from build123d import *

# Parameters (mm, degrees)
SKETCH1_W           = 22
SKETCH1_H           = 20
BOSS_EXTRUDE1_DEPTH = 18
SKETCH2_W           = 12
SKETCH2_H           = 8
CUT_EXTRUDE1_DEPTH  = 15
SKETCH3_W           = 18
SKETCH3_H           = 5
BOSS_EXTRUDE2_DEPTH = 2
LPATTERN1_COUNT     = 6
LPATTERN1_PITCH     = 24
SKETCH4_W           = 18
SKETCH4_H           = 15
BOSS_EXTRUDE3_DEPTH = 2
SKETCH5_W           = 18
SKETCH5_H           = 20
BOSS_EXTRUDE4_DEPTH = 2
SKETCH6_W           = 132
SKETCH6_H           = 2
CUT_EXTRUDE2_DEPTH  = 2
SKETCH7_W           = 146
SKETCH7_H           = 18
BOSS_EXTRUDE5_DEPTH = 6


with BuildPart() as part:
    # Sketch1 → Boss-Extrude1 (new body)
    with BuildSketch(Plane.XY):
        with Locations((11, 10)):
            Rectangle(SKETCH1_W, SKETCH1_H)
    extrude(amount=BOSS_EXTRUDE1_DEPTH)

    # Sketch2 → Cut-Extrude1 (cut)
    with BuildSketch(Plane.XZ):
        with Locations((11, 9)):
            Rectangle(SKETCH2_W, SKETCH2_H)
    extrude(amount=-CUT_EXTRUDE1_DEPTH, mode=Mode.SUBTRACT)

    # Sketch3 → Boss-Extrude2 (add)
    with BuildSketch(Plane(origin=(22, 0, 0), x_dir=(0, 0, -1), z_dir=(1, 0, 0))):
        with Locations((-9, 2.5)):
            Rectangle(SKETCH3_W, SKETCH3_H)
    extrude(amount=BOSS_EXTRUDE2_DEPTH)


with BuildPart() as lpattern1_1:
    # LPattern1: pattern copy
    add(part.part.moved(Location(Vector(1, 0, 0) * (1 * LPATTERN1_PITCH))))


with BuildPart() as lpattern1_2:
    # LPattern1: pattern copy
    add(part.part.moved(Location(Vector(1, 0, 0) * (2 * LPATTERN1_PITCH))))


with BuildPart() as lpattern1_3:
    # LPattern1: pattern copy
    add(part.part.moved(Location(Vector(1, 0, 0) * (3 * LPATTERN1_PITCH))))


with BuildPart() as lpattern1_4:
    # LPattern1: pattern copy
    add(part.part.moved(Location(Vector(1, 0, 0) * (4 * LPATTERN1_PITCH))))


with BuildPart() as lpattern1_5:
    # LPattern1: pattern copy
    add(part.part.moved(Location(Vector(1, 0, 0) * (5 * LPATTERN1_PITCH))))


with BuildPart() as lpattern1_2_1:
    add(lpattern1_2.part)

    # Combine1: union part, LPattern1_3, LPattern1_4, LPattern1_5, LPattern1_1
    add(part.part)
    add(lpattern1_3.part)
    add(lpattern1_4.part)
    add(lpattern1_5.part)
    add(lpattern1_1.part)

    # Sketch4 → Boss-Extrude3 (add)
    with BuildSketch(Plane(origin=(142, 0, 0), x_dir=(0, 0, -1), z_dir=(1, 0, 0))):
        with Locations((-9, 12.5)):
            Rectangle(SKETCH4_W, SKETCH4_H)
    extrude(amount=BOSS_EXTRUDE3_DEPTH)

    # Sketch5 → Boss-Extrude4 (add)
    with BuildSketch(Plane.ZY):
        with Locations((9, 10)):
            Rectangle(SKETCH5_W, SKETCH5_H)
    extrude(amount=BOSS_EXTRUDE4_DEPTH)

    # Sketch6 → Cut-Extrude2 (cut)
    with BuildSketch(Plane(origin=(0, 0, 0), x_dir=(-1, 0, 0), z_dir=(0, -1, 0))):
        with Locations((-71, -9)):
            Rectangle(SKETCH6_W, SKETCH6_H)
    extrude(amount=-CUT_EXTRUDE2_DEPTH, mode=Mode.SUBTRACT)

    # Sketch7 → Boss-Extrude5 (add)
    with BuildSketch(Plane.XZ):
        with Locations((71, 9)):
            Rectangle(SKETCH7_W, SKETCH7_H)
    extrude(amount=BOSS_EXTRUDE5_DEPTH)


solid = lpattern1_2_1.part
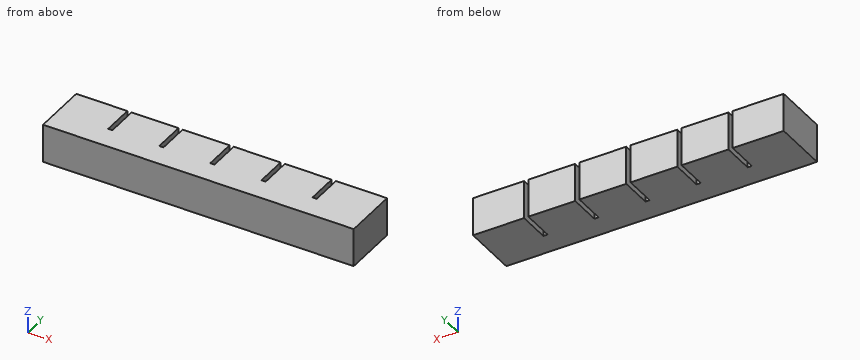
Geometry: final body of the model. Coordinates: model frame, mm. Coordinates: 2 decimals unless noted, no trailing zeros. Loops run counter-clockwise (first coordinate to the right, second up) from the corner with the lowest first, then second, coordinate; pieces in that order, holes last. Notation, with made-up numbers: (-19.75, -12.75) - (14.25, -12.75) arc R20 cw to (14.25, 8.25) - close; hole circle Ø9 at (53.5, 81.5). An arc over 180 degrees is marked (long way). Put each result on its own line as item: value. Start each with the question number.
Q1. Cut plane A-A, the plane x = 32. Return loops of the section in (y, z), and give its area (3 significant figures).
Q2. Cut plane B-B, the plane z = 15. Return loops of the section in (x, y).
Q3. Pin query (flat end, axial travel): pin 1 Ø1 at (x, z) = (71, 5.5) entering from +Y. Return the tip coordinate at first contact, or that it passes through.
Q4. Line query: line 1 (X direction, y = 12.75, z = 4.25); line 2 (Y direction, x = 68, z = 8.5); line 3 (Z direction, x = 63.5, y = 13.5). Output: solid intervals per line, ascending.
Q5. Cut plane C-C, the plane y = 10.75. Give the number of separate pieces and of enclosed holes in the cut face, and give its area (3 significant figures).
Filled sheet:
1. outline: (-6, 0) - (20, 0) - (20, 18) - (-6, 18) - close; hole (0, 5) - (15, 5) - (15, 13) - (0, 13) - close
1. area: 348 mm²
2. outline: (-2, -6) - (144, -6) - (144, 20) - (120, 20) - (120, 5) - (118, 5) - (118, 20) - (96, 20) - (96, 5) - (94, 5) - (94, 20) - (72, 20) - (72, 5) - (70, 5) - (70, 20) - (48, 20) - (48, 5) - (46, 5) - (46, 20) - (24, 20) - (24, 5) - (22, 5) - (22, 20) - (-2, 20) - close
3. pin 1: y = 5
4. line 1: -2 to 22, 24 to 46, 48 to 70, 72 to 94, 96 to 118, 120 to 144
4. line 2: -6 to 0, 2 to 20
4. line 3: 0 to 5, 13 to 18
5. separate pieces: 6
5. enclosed holes: 6
5. area: 1,870 mm²
